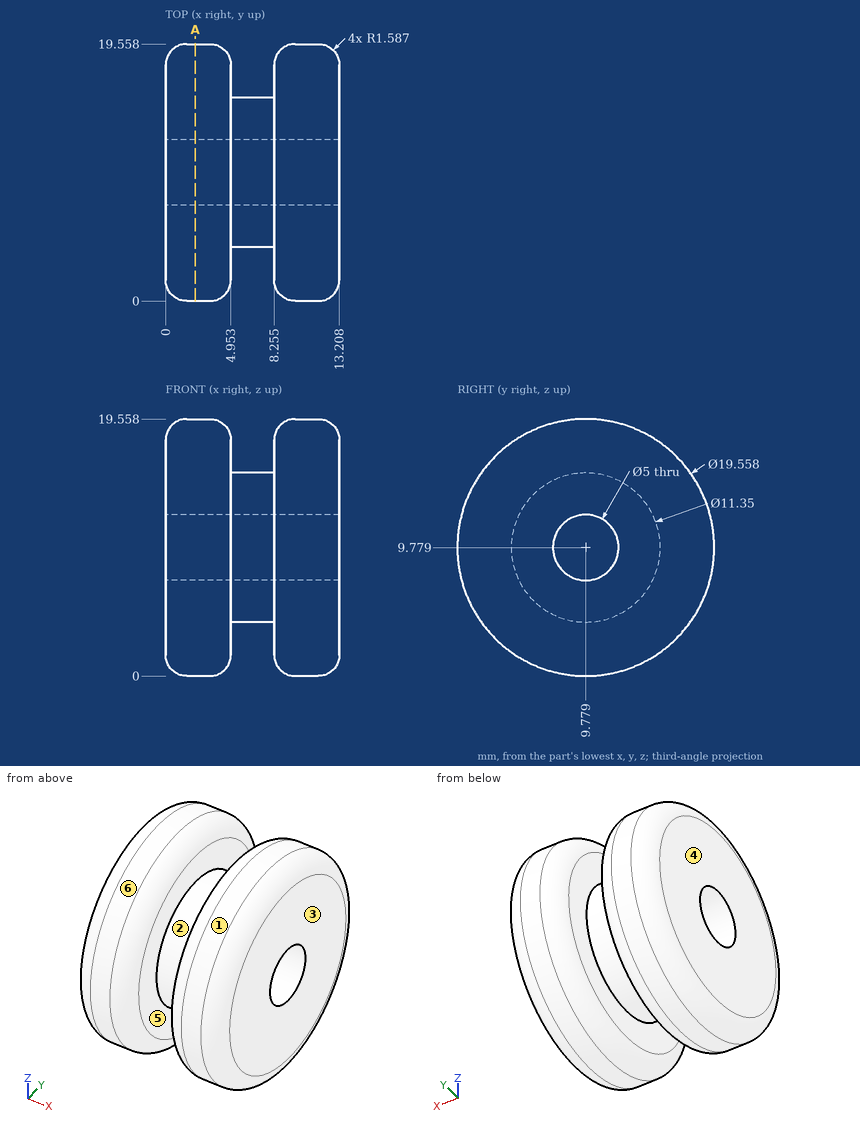
Here's the drawing with two shaded views (mm, measured from the low corner). I have some questions. A direction names the side the tool comes from. Give positions to 0.01 mm unless a question says otherwise; leave off trailing zeros. Order: outer loops, then holes, each group sorted by start corner. A loop starts at its lowest first (then second) coordinate and runs counter-clockwise, first axis right, second up. Notation, with made-up numbers: M 8,42.25 L 12,42.25 A5 cw 12,47.25 Z; hole C -33,2.5 d10. An arc over 180 degrees is marked long. Answer as a JSON object with one key per item and string values. Group by question number.
1) Suppose I cut it at A-A, the plane x = 2.25. Write out the boundary of the cut face in (y, z), plus the area to 3 significant figures.
2) On a 3-axis mill with a long thin cutter (end or side, diameter ignored), from which of +Z, -Z, +X, -X, +Y, -Y can I reach the whole of each face in a straight line? I mean the marked faces 5 and 6. Say none if no direction works.
3) Please list where these lines run through material, in increasing order: L1, parallel to X at y = 4, z = 9 (1 decimal); L2, parallel to Y at x = 7.5, z = 9 (1 decimal); L3, parallel to Z at x = 12.5, y = 7.75 (1 decimal). Write a range as [from, to].
4) I'm going to push flat-ended pins straight in: pin 1 Ø2 at (x, z) = (4.5, 14.5) entering from +Y; pin 2 Ø4 at (x, z) = (5.5, 9.5) entering from +Y; pin 3 Ø4 at (x, z) = (5.5, 14.5) entering from -Y. Where does each tip first touch, or does it pass through?
5) We'd pull the mould along X, two halves only. Please class the marked faces 1, 2, 3 and 4: pulls with the +X half, pulls with the -X half, needs draft (parallel to the pull), parting line crosses it, or undercut.
Results found:
{
 "1": {"outline": "C 9.78,9.78 d19.56; hole C 9.78,9.78 d5", "area": "281 mm²"},
 "2": {"face 5": "none", "face 6": "+X, -X"},
 "3": {"L1": "[0, 5], [8.3, 13.2]", "L2": "[4.2, 7.4], [12.2, 15.4]", "L3": "[0.5, 8.3], [11.2, 19.1]"},
 "4": {"pin 1": "y = 18.64", "pin 2": "y = 19.55", "pin 3": "y = 0.75"},
 "5": {"face 1": "needs draft", "face 2": "undercut", "face 3": "pulls with the +X half", "face 4": "pulls with the -X half"}
}
